Build history of the part. All positions in model axes, mm. A direction names the side the tool comes from. Give positions to 0.01 mm unless a question says otherwise; leave off trailing zeros. Order: outer loops, then holes, each group sorted by start corner. A loop starts at its lowest first (then second) coordinate and runs counter-clockwise, first axis right, second up. Notation, with made-up numbers: M -19.75,19.25 L -5.75,19.25 A23 cw -5.75,38.25 Z; hole C 44.5,-32.5 d9. An arc over 180 degrees is marked long. One line per item, written item: value.
from build123d import *

# Parameters (mm, degrees)
BOSS_EXTRUDE10_DEPTH = 2
BOSS_EXTRUDE11_DEPTH = 1.5
SKETCH8_R            = 1.5
BOSS_EXTRUDE12_DEPTH = 21


with BuildPart() as part:
    # Sketch1 → Boss-Extrude10 (new body)
    with BuildSketch(Plane.XY):
        with BuildLine():
            ThreePointArc((2.5, 18.834808202), (0, 19), (-2.5, 18.834808202))
            Line((-2.5, 18.834808202), (-2.5, 18.653696235))
            Line((-2.5, 18.653696235), (2.5, 18.653696235))
            Line((2.5, 18.653696235), (2.5, 18.834808202))
        make_face()
        with BuildLine():
            Line((-2.5, 23.653696235), (-2.5, 18.834808202))
            ThreePointArc((-2.5, 18.834808202), (0, 19), (2.5, 18.834808202))
            Line((2.5, 18.834808202), (2.5, 23.653696235))
            Line((2.5, 23.653696235), (-2.5, 23.653696235))
        make_face()
        with BuildLine():
            ThreePointArc((-2.5, 18.834808202), (-14.123191749, 12.709659901), (-18.993227641, 0.507251182))
            Line((-18.993227641, 0.507251182), (-17.892811301, 0.507251182))
            ThreePointArc((-17.892811301, 0.507251182), (0, 17.9), (17.892811301, 0.507251182))
            Line((17.892811301, 0.507251182), (18.993227641, 0.507251182))
            ThreePointArc((18.993227641, 0.507251182), (14.123191749, 12.709659901), (2.5, 18.834808202))
            Line((2.5, 18.834808202), (2.5, 18.653696235))
            Line((2.5, 18.653696235), (-2.5, 18.653696235))
            Line((-2.5, 18.653696235), (-2.5, 18.834808202))
        make_face()
        with BuildLine():
            Line((-17.893216553, -0.492748818), (-18.993609415, -0.492748818))
            ThreePointArc((-18.993609415, -0.492748818), (-14.12804293, -12.704267117), (-2.5, -18.834808202))
            Line((-2.5, -18.834808202), (-2.5, -18.60362099))
            Line((-2.5, -18.60362099), (2.384110391, -18.60362099))
            Line((2.384110391, -18.60362099), (2.384110391, -18.849828053))
            ThreePointArc((2.384110391, -18.849828053), (14.088907535, -12.747654077), (18.993609415, -0.492748818))
            Line((18.993609415, -0.492748818), (17.893216553, -0.492748818))
            ThreePointArc((17.893216553, -0.492748818), (0, -17.9), (-17.893216553, -0.492748818))
        make_face()
        with BuildLine():
            Line((10.988958031, -0.492748818), (-10.988958031, -0.492748818))
            ThreePointArc((-10.988958031, -0.492748818), (0, -11), (10.988958031, -0.492748818))
        make_face()
        with BuildLine():
            Line((10.98829815, 0.507251182), (-10.98829815, 0.507251182))
            ThreePointArc((-10.98829815, 0.507251182), (-10.999997605, 0.007258684), (-10.988958031, -0.492748818))
            Line((-10.988958031, -0.492748818), (10.988958031, -0.492748818))
            ThreePointArc((10.988958031, -0.492748818), (10.997239161, -0.246436261), (11, 0))
            ThreePointArc((11, 0), (10.997074148, 0.25369307), (10.98829815, 0.507251182))
        make_face()
        with BuildLine():
            ThreePointArc((10.98829815, 0.507251182), (0, 11), (-10.98829815, 0.507251182))
            Line((-10.98829815, 0.507251182), (10.98829815, 0.507251182))
        make_face()
        with BuildLine():
            ThreePointArc((2.384110391, -18.849828053), (-0.058429439, -18.999910158), (-2.5, -18.834808202))
            Line((-2.5, -18.834808202), (-2.5, -23.60362099))
            Line((-2.5, -23.60362099), (2.384110391, -23.60362099))
            Line((2.384110391, -23.60362099), (2.384110391, -18.849828053))
        make_face()
        with BuildLine():
            Line((-2.5, -18.60362099), (-2.5, -18.834808202))
            ThreePointArc((-2.5, -18.834808202), (-0.058429439, -18.999910158), (2.384110391, -18.849828053))
            Line((2.384110391, -18.849828053), (2.384110391, -18.60362099))
            Line((2.384110391, -18.60362099), (-2.5, -18.60362099))
        make_face()
    extrude(amount=BOSS_EXTRUDE10_DEPTH)

    # Sketch7 → Boss-Extrude11 (add, symmetric)
    with BuildSketch(Plane(origin=(0, 0, 0), x_dir=(0, 0, -1), z_dir=(1, 0, 0))):
        with BuildLine():
            ThreePointArc((0, 21.244252218), (21.23548837, 0.008763848), (0, -21.226724522))
            Line((0, -21.226724522), (0, -23.60362099))
            ThreePointArc((0, -23.60362099), (23.628658612, 0.025037622), (0, 23.653696235))
            Line((0, 23.653696235), (0, 21.244252218))
        make_face()
        with BuildLine():
            ThreePointArc((18.174866248, -10.973959092), (21.23548837, 0.008763848), (18.174866248, 10.991486788))
            Line((18.174866248, 10.991486788), (18.174866248, -10.973959092))
        make_face()
    extrude(amount=BOSS_EXTRUDE11_DEPTH, both=True)

    # Sketch8 → Boss-Extrude12 (add)
    with BuildSketch(Plane.XY):
        Circle(SKETCH8_R)
    extrude(amount=-BOSS_EXTRUDE12_DEPTH)


solid = part.part
1) Saw through at D-D, the plane y = 14. Write the cut outline in (x, z).
Check values:
outline: M -12.85,0 L -11.15,0 L -11.15,2 L -12.85,2 Z; M -1.5,-19.05 L 1.5,-19.05 L 1.5,-15.97 L -1.5,-15.97 Z; M 11.15,0 L 12.85,0 L 12.85,2 L 11.15,2 Z
2) Pin check, flat tips, straight feed: pin 1 (1.6 mm diameter, centred on y = 20.5, z = 1, fed in from +X); pin 2 (18.5 mm diameter, centred on x = -3, y = -8.5, fed in from -Z); pin 3 (1 mm diameter, centred on y = -22, z = 0.5, fed in from -X); pin 4 (6 mm diameter, centred on y = 6.5, z = -9, fed in from -X). Stop position of each tip, or through.
Check values:
pin 1: x = 2.5
pin 2: z = -23.63
pin 3: x = -2.5
pin 4: through
3) Saw through at C-C, the plane y = 19.5. Write the cut outline in (x, z), then the cut area to 3 significant figures.
Check values:
outline: M -2.5,0 L 2.5,0 L 2.5,2 L -2.5,2 Z; M -1.5,-13.38 L 1.5,-13.38 L 1.5,-8.43 L -1.5,-8.43 Z
area: 24.9 mm^2
4) Saw through at B-B, the plane x = 9. Write the cut outline in (y, z).
Check values:
outline: M -16.73,0 L -15.47,0 L -15.47,2 L -16.73,2 Z; M -6.32,0 L 6.32,0 L 6.32,2 L -6.32,2 Z; M 15.47,0 L 16.73,0 L 16.73,2 L 15.47,2 Z
5) Drill centre lines: probe 1 along Y at (x, z) = (-1, -1.25); probe 2 along Y at (x, z) = (1, -17.25); probe 3 along Z at (x, y) = (11, -14.5). Where is each one in solid material? Low to high. Write a range as from..to.
Check values:
probe 1: -23.57..-21.19, -1.12..1.12, 21.21..23.62
probe 2: -16.12..-12.38, -1.12..1.12, 12.39..16.17
probe 3: 0..2
6) Saw through at A-A, the plane z = -6.25. Write the cut outline in (x, y).
Check values:
outline: M -1.5,-22.76 L 1.5,-22.76 L 1.5,-20.29 L -1.5,-20.29 Z; C 0,0 d3; M -1.5,20.3 L 1.5,20.3 L 1.5,22.81 L -1.5,22.81 Z
7) Tool access for faces 1 (the face through (-2.5, -21, 1)), 2 (the face through (0.02, -18.41, -10.57)), 3 (the face through (-18.5, 0.507, 1)): list every direction of +Z, -Z, +X, -X, +Y, -Y with a clear straight run to the whole face (end or side of a thin tool).
Check values:
face 1: +Z, -Z, -X, -Y
face 2: +X, -X
face 3: +Z, -Z, -X
8) Mould opens along X. For faces 4 (the face through (-0.387, 17.896, 0.986)), 5 (the face through (-14.253, -12.564, 0.986)), 6 (the face through (2, 0, 0)) say: released by +X, released by -X, zero draft, split by the parting line, or undercut.
Check values:
face 4: undercut
face 5: released by -X
face 6: zero draft
